Geometry: see drawing. Coordinates: mm, zero at the bounding-box minimum. A direction names the side the tool comes from. Round coordinates to 2 decimals unless told otherwise and drop trailing zeros. Loops run counter-clockwise (first coordinate to the right, second up) from the corner with the lowest first, then second, coordinate; pieces in that order, holes last. Notation, with made-up numbers: M 23,-20 L 78,-20 A26 ccw 78,15 Z; hole C -8.5,53.25 d1. An arc over 180 degrees is marked long. Answer as a JSON object with one key per item and string values.
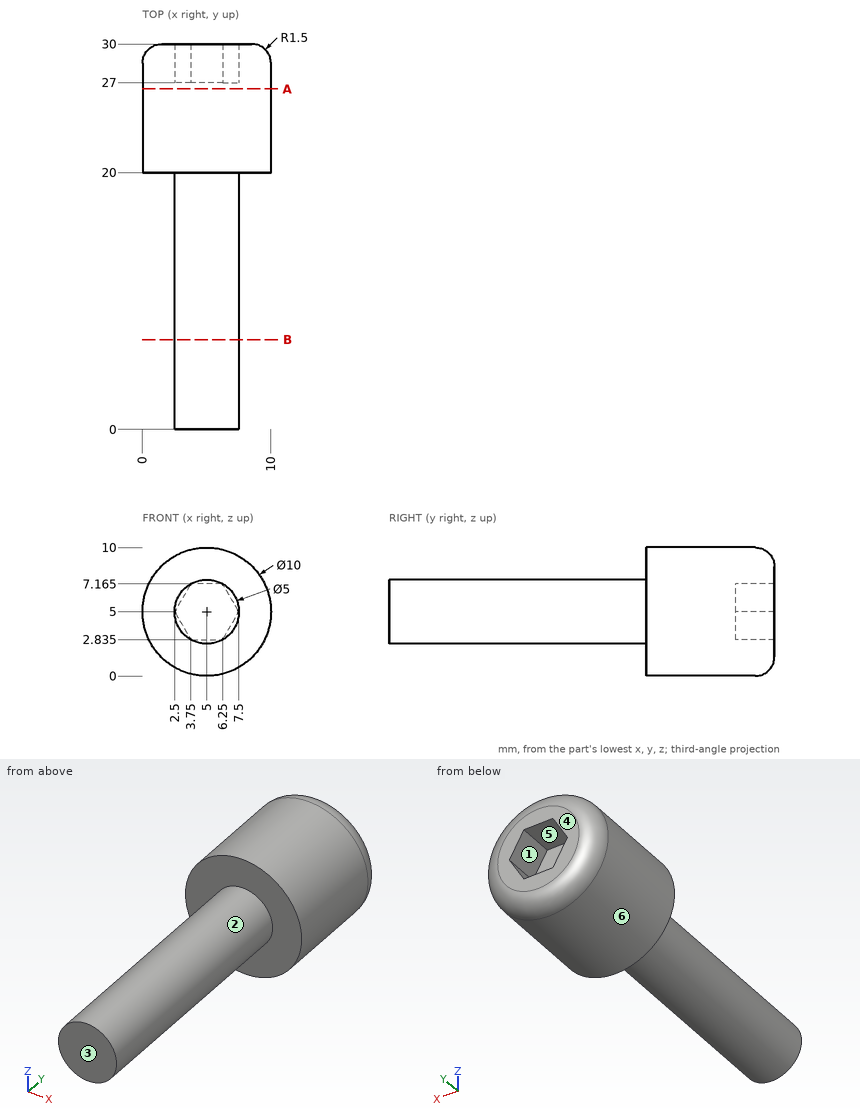
1) Pin query (flat end, axial travel): P1, Ø1.2, axis at x = 5.5, y = 29, coming from the -Z side; P2, Ø1, axis at y = 10, z = 4, coming from the +X side; P3, Ø0.8, axis at x = 5, y = 29, coming from the +Z side. Return the tip coordinate at first contact, or that it passes through.
Results:
{"P1": "z = 0", "P2": "x = 7.45", "P3": "z = 10"}
2) Section query A-A (y = 26.5). Return the cut outline in (x, z), and give its area (3 significant figures).
Results:
{"outline": "C 5,5 d10", "area": "78.5 mm2"}
3) Section query B-B (y = 7). Return the cut outline in (x, z).
Results:
{"outline": "C 5,5 d5"}
4) Pull-direction query (X, two-part tool) for the marked faces 4, 5 and 6; classes: +X half, -X half, draft (parallel to the pull), parting line (faces both ways), or undercut.
Results:
{"face 4": "draft", "face 5": "undercut", "face 6": "parting line"}
5) Ray query, line 1 (Y direction, x = 7.75, z = 5.5); line 2 (X direction, y = 11, z = 6.75) (1 decimal); line 3 (Z direction, x = 4.5, y = 27.5) (3 decimals). Return the intervals inside material, ascending.
Results:
{"line 1": "20 to 30", "line 2": "3.2 to 6.8", "line 3": "0.025 to 2.835, 7.165 to 9.975"}
6) Reachability of the marked faces 1, 2 and 3 from +Z, -Z, +X, -X, +Y, -Y: full face, straight path, thin tool, end or side. Return the list, or none.
Results:
{"face 1": "+Y", "face 2": "-Y", "face 3": "+Z, -Z, +X, -X, -Y"}
